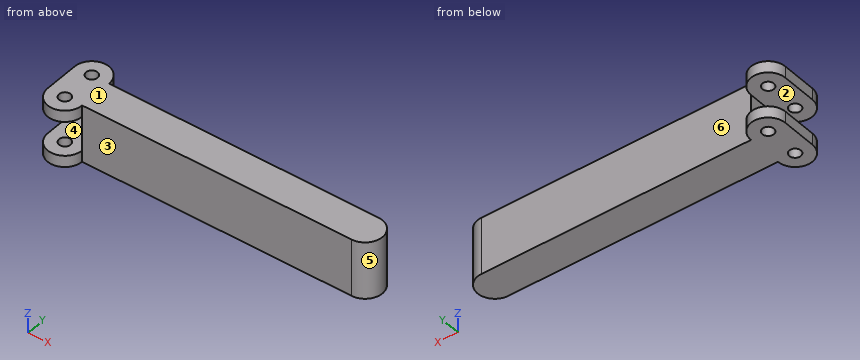
```python
from build123d import *

# Parameters (mm, degrees)
SKETCH1_R           = 3.175
BOSS_EXTRUDE1_DEPTH = 31.75
SKETCH6_W           = 19.05
SKETCH6_H           = 19.05
SKETCH6_H_2         = 9.525
CUT_EXTRUDE1_DEPTH  = 19.05


with BuildPart() as part:
    # Sketch1 → Boss-Extrude1 (new body)
    with BuildSketch(Plane.XY):
        with BuildLine():
            Line((-9.525, 0), (-9.525, 19.05))
            ThreePointArc((-9.525, 19.05), (0, 28.575), (9.525, 19.05))
            Line((9.525, 19.05), (158.75, 19.05))
            ThreePointArc((158.75, 19.05), (168.275, 9.525), (158.75, 0))
            Line((158.75, 0), (9.525, 0))
            ThreePointArc((9.525, 0), (0, -9.525), (-9.525, 0))
        make_face()
        with Locations((0, 19.05)):
            Circle(SKETCH1_R, mode=Mode.SUBTRACT)
        Circle(SKETCH1_R, mode=Mode.SUBTRACT)
    extrude(amount=BOSS_EXTRUDE1_DEPTH)

    # Sketch6 → Cut-Extrude1 (cut)
    with BuildSketch(Plane.ZY.offset(9.525)):
        with Locations((15.875, 9.525)):
            Rectangle(SKETCH6_W, SKETCH6_H)
        with Locations((15.875, 23.8125)):
            Rectangle(SKETCH6_W, SKETCH6_H_2)
        with Locations((15.875, -4.7625)):
            Rectangle(SKETCH6_W, SKETCH6_H_2)
    extrude(amount=-CUT_EXTRUDE1_DEPTH, mode=Mode.SUBTRACT)


solid = part.part
```
The listing builds one solid part. Answer for the finished solid, in the listing's coordinates (mm). Face numbers are marked on the shaded views. A direction names the side the tool comes from. Give positions to 0.01 mm unless a question says otherwise; leave off trailing zeros. Write each loop counter-clockwise with the first axis right and the second up, starting at its lowest first coordinate (ties: lowest second). Pieces come first, ordered by that corner, then holes. Notation, with made-up numbers: (63.25, 48) -> (112.25, 48) arc R24 cw to (112.25, 75) -> close; hole circle Ø3 at (16.25, 72). An arc over 180 degrees is marked (long way). Use one line per item in the form item = value.
1) For a pull along Z with two mould halves and no side action, classify the marked faces 1, 2, 3 and 4 as +Z half, -Z half, draft (parallel to the pull), parting line (faces both ways), or undercut.
Result:
face_1 = +Z half
face_2 = undercut
face_3 = draft
face_4 = undercut
2) Section C-C on y = 10.5 is taken. Write down the section's boundary in (x, z) (3 decimals), plus the area to 3 significant figures.
Result:
outline = (-9.525, 0) -> (168.225, 0) -> (168.225, 31.75) -> (-9.525, 31.75) -> (-9.525, 25.4) -> (9.525, 25.4) -> (9.525, 6.35) -> (-9.525, 6.35) -> close
area = 5,280 mm²
3) Section A-A on x = 0 is taken. Write down the section's boundary in (y, z) (3 decimals), plus the area to 3 significant figures.
Result:
outline = (-9.525, 0) -> (-3.175, 0) -> (-3.175, 6.35) -> (-9.525, 6.35) -> close; (-9.525, 25.4) -> (-3.175, 25.4) -> (-3.175, 31.75) -> (-9.525, 31.75) -> close; (3.175, 0) -> (15.875, 0) -> (15.875, 6.35) -> (3.175, 6.35) -> close; (3.175, 25.4) -> (15.875, 25.4) -> (15.875, 31.75) -> (3.175, 31.75) -> close; (22.225, 0) -> (28.575, 0) -> (28.575, 6.35) -> (22.225, 6.35) -> close; (22.225, 25.4) -> (28.575, 25.4) -> (28.575, 31.75) -> (22.225, 31.75) -> close
area = 323 mm²
4) Each of these flat-tipped pins is pushed along its axis until it touches: P1, Ø10, axis at x = 0, y = 0, coming from the -Z side; P2, Ø9.5, axis at y = 6.5, z = 12.5, coming from the -X side (3 decimals); P3, Ø9.5, axis at x = 104.5, z = 8.5, coming from the -Y side; P4, Ø2, axis at y = 4, z = 24, coming from the +X side. Where does it stop, or does it pass through?
Result:
P1 = 0
P2 = 9.525
P3 = 0
P4 = 167.13
5) A tool of negligible diameter and unlimited length cuts with its end or side. For the marked faces 5 and 6, from which of +Z, -Z, +X, -X, +Y, -Y can it reach the whole face along a straight path? Write none if from no direction.
Result:
face_5 = +Z, -Z, +X
face_6 = +Z, -Z, +X, +Y
6) Section B-B on x = 55.5 is taken. Write down the section's boundary in (y, z), plus the area to 3 significant figures.
Result:
outline = (0, 0) -> (19.05, 0) -> (19.05, 31.75) -> (0, 31.75) -> close
area = 605 mm²
7) Straight lines are drawn through the part: probe 1 along Y at (x, z) = (0, 29) (3 decimals); probe 2 along Z at (x, y) = (4, 24); probe 3 along Y at (x, z) = (153, 15). For each, find the intervals that lie inside material, in ascending order.
Result:
probe_1 = -9.525 to -3.175, 3.175 to 15.875, 22.225 to 28.575
probe_2 = 0 to 6.35, 25.4 to 31.75
probe_3 = 0 to 19.05
